The listing builds one solid part. Answer for the finished solid, in the listing's coordinates (mm). A direction names the side the tool comes from. Give positions to 0.01 mm unless a question says otherwise; leave off trailing zeros. Write each loop counter-clockwise with the first axis right and the second up, starting at its lowest first coordinate (ties: lowest second). Pieces come first, ordered by that corner, then holes.
```python
from build123d import *

# Parameters (mm, degrees)
BOSS_EXTRU_1_DEPTH           = 1
BOSS_EXTRU_2_DEPTH           = 20
ENL_V_MAT_EXTRU_1_DEPTH      = 51.671873049
ENL_V_MAT_EXTRU_1_DEPTH_BACK = 51.671873049
ESQUISSE5_W                  = 1.5
ESQUISSE5_H                  = 5
ESQUISSE9_W                  = 10
ESQUISSE9_H                  = 3
BOSS_EXTRU_5_DEPTH           = 1
CONG_1_R                     = 0.5
ESQUISSE10_W                 = 10
ESQUISSE10_H                 = 3
BOSS_EXTRU_6_DEPTH           = 1
CONG_2_R                     = 0.5


with BuildPart() as part:
    # Esquisse1 → Boss.-Extru.1 (new body)
    with BuildSketch(Plane.XY):
        Polygon((34.845351237, 9.251363312), (-20.154648763, 9.251363312), (-30.154648763, -0.748636688), (-20.154648763, -10.748636688), (34.845351237, -10.748636688), (44.845351237, -0.748636688), align=None)
    extrude(amount=BOSS_EXTRU_1_DEPTH)

    # Esquisse2 → Boss.-Extru.2 (add)
    with BuildSketch(Plane.XY.offset(1)):
        Polygon((-20.154648763, -10.748636688), (34.845351237, -10.748636688), (44.845351237, -0.748636688), (34.845351237, 9.251363312), (-20.154648763, 9.251363312), (-30.154648763, -0.748636688), align=None)
        Polygon((-19.491907063, 7.651363312), (-27.891907063, -0.748636688), (-19.491907063, -9.148636688), (34.182609538, -9.148636688), (42.582609538, -0.748636688), (34.182609538, 7.651363312), align=None, mode=Mode.SUBTRACT)
    extrude(amount=BOSS_EXTRU_2_DEPTH)

    # Esquisse5 → Enlèv. mat.-Extru.1 (cut, two sides: drawn at the far end of the back side and taken through both)
    with BuildSketch(Plane(origin=(0, 0, 0), x_dir=(0, 0, -1), z_dir=(1, 0, 0)).offset(-ENL_V_MAT_EXTRU_1_DEPTH_BACK)):
        with Locations((-2.25, -0.748636688)):
            Rectangle(ESQUISSE5_W, ESQUISSE5_H)
    extrude(amount=ENL_V_MAT_EXTRU_1_DEPTH + ENL_V_MAT_EXTRU_1_DEPTH_BACK, mode=Mode.SUBTRACT)

    # Esquisse9 → Boss.-Extru.5 (add)
    with BuildSketch(Plane(origin=(0, 9.251363312, 0), x_dir=(1, 0, 0), z_dir=(0, 1, 0))):
        with Locations((7.345351237, -14.5)):
            Rectangle(ESQUISSE9_W, ESQUISSE9_H)
    extrude(amount=BOSS_EXTRU_5_DEPTH)

    # Congé1
    cong_1_edges = [part.edges().sort_by_distance(p)[0] for p in [
        (2.345351237, 10.251363312, 14.5),
        (7.345351237, 10.251363312, 16),
        (12.345351237, 10.251363312, 14.5),
        (7.345351237, 10.251363312, 13),
    ]]
    fillet(cong_1_edges, radius=CONG_1_R)

    # Esquisse10 → Boss.-Extru.6 (add)
    with BuildSketch(Plane.XZ.offset(10.748636688)):
        with Locations((7.345351237, 14.5)):
            Rectangle(ESQUISSE10_W, ESQUISSE10_H)
    extrude(amount=BOSS_EXTRU_6_DEPTH)

    # Congé2
    cong_2_edges = [part.edges().sort_by_distance(p)[0] for p in [
        (2.345351237, -11.748636688, 14.5),
        (7.345351237, -11.748636688, 13),
        (12.345351237, -11.748636688, 14.5),
        (7.345351237, -11.748636688, 16),
    ]]
    fillet(cong_2_edges, radius=CONG_2_R)


solid = part.part
```
Item 1: Which of the six approach directions +Z, -Z, +X, -X, +Y, -Y give full straight-line access (tool end or side, diameter ignored) to faces 1 (the face through (-28, -1, 1.5)), 2 (the face through (7, 10.251, 14)), 3 (the face through (38.441, 3.393, 10.86))?
Conclusion:
face 1: +X, -X
face 2: +Z, -Z, +X, -X, +Y
face 3: +Z
Item 2: A cutting plane is placed at C-C, the plane z = 7.5. Give the vertices of the cut face in (x, y).
Conclusion:
outline: (-30.15, -0.75) - (-20.15, -10.75) - (34.85, -10.75) - (44.85, -0.75) - (34.85, 9.25) - (-20.15, 9.25) - close; hole (-27.89, -0.75) - (-19.49, -9.15) - (34.18, -9.15) - (42.58, -0.75) - (34.18, 7.65) - (-19.49, 7.65) - close
Item 3: Determine the mould class of faces 4 (the face through (8, 7.651, 11)), 5 (the face through (41, 1.751, 2)), 6 (the face through (39.915, 4.181, 10.353)), 7 (the face through (-23.75, -4.89, 10.86)) for opening direction X: pulls with the +X half, pulls with the -X half, needs draft (parallel to the pull), parting line crosses it, or undercut.
Conclusion:
face 4: undercut
face 5: needs draft
face 6: pulls with the +X half
face 7: undercut
Item 4: Consider probe 1 along Y at (x, z) = (6, 3); probe 2 along Y at (x, z) = (6.5, 14.5); probe 3 along Z at (x, y) = (15, -3). Determine where each line is inside the solid, lowest interval first.
Conclusion:
probe 1: y = -10.75 to -9.15, 7.65 to 9.25
probe 2: y = -11.75 to -9.15, 7.65 to 10.25
probe 3: z = 0 to 1
Item 5: A cutting plane is placed at D-D, the plane y = 4.5. Give the vertices of the cut face in (x, z), plus the area to 3 significant figures.
Conclusion:
outline: (-24.91, 0) - (39.6, 0) - (39.6, 21) - (37.33, 21) - (37.33, 1) - (-22.64, 1) - (-22.64, 21) - (-24.91, 21) - close
area: 155 mm2
Item 6: Each of these flat-tipped pins is pushed along its axis until it touches: P1, Ø1, axis at x = 12, y = 6.5, coming from the +Z side; P2, Ø0.8, axis at x = -27, z = 2.5, coming from the +Y side; P3, Ø6.5, axis at x = -1.5, z = 14, coming from the +Y side; P4, Ø1, axis at x = -14.5, y = -5.5, coming from the -Z side. Where does it stop, or does it pass through?
Conclusion:
P1: stops at z = 1
P2: stops at y = 2.81
P3: stops at y = 9.25
P4: stops at z = 0
Item 7: A cutting plane is placed at B-B, the plane x = -7. Give the vertices of the cut face in (y, z).
Conclusion:
outline: (-10.75, 0) - (9.25, 0) - (9.25, 21) - (7.65, 21) - (7.65, 1) - (-9.15, 1) - (-9.15, 21) - (-10.75, 21) - close
Item 8: A cutting plane is placed at A-A, the plane z = 2.25. Give the vertices of the cut face in (x, y).
Conclusion:
outline: (-27.65, -3.25) - (-20.15, -10.75) - (34.85, -10.75) - (42.35, -3.25) - (40.08, -3.25) - (34.18, -9.15) - (-19.49, -9.15) - (-25.39, -3.25) - close; (-27.65, 1.75) - (-25.39, 1.75) - (-19.49, 7.65) - (34.18, 7.65) - (40.08, 1.75) - (42.35, 1.75) - (34.85, 9.25) - (-20.15, 9.25) - close
